```python
from build123d import *

# Parameters (mm, degrees)
SKETCH2_R           = 9.7
SKETCH2_R_2         = 6.75
SKETCH2_W           = 4.5
SKETCH2_H           = 14.8
SKETCH2_W_2         = 16.6
SKETCH2_H_2         = 4.4
BOSS_EXTRUDE1_DEPTH = 3.7
FILLET1_R           = 15
FILLET2_R           = 25
FILLET3_R           = 10


with BuildPart() as part:
    # Sketch2 → Boss-Extrude1 (new body)
    with BuildSketch(Plane.XY):
        Polygon((-66.408376963, -37.473298429), (-66.408376963, 53.126701571), (-57.108376963, 53.126701571), (-39.206701064, 34.826701571), (48.193298936, 34.826701571), (65.490462758, 53.699118578), (74.790462758, 53.699118578), (74.790462758, -29.400881422), align=None)
        with Locations((55.690462758, -8.957731732)):
            Circle(SKETCH2_R, mode=Mode.SUBTRACT)
        with Locations((-42.158376963, -6.98947646)):
            Circle(SKETCH2_R_2, mode=Mode.SUBTRACT)
        with Locations((-60.558376963, 35.726701571)):
            Rectangle(SKETCH2_W, SKETCH2_H, mode=Mode.SUBTRACT)
        with Locations((70.815419874, 35.726701571)):
            Rectangle(SKETCH2_W, SKETCH2_H, mode=Mode.SUBTRACT)
        with Locations((-11.433419848, 23.626701571)):
            Rectangle(SKETCH2_W_2, SKETCH2_H_2, mode=Mode.SUBTRACT)
        with Locations((21.690462758, 23.626701571)):
            Rectangle(SKETCH2_W_2, SKETCH2_H_2, mode=Mode.SUBTRACT)
        with BuildLine():
            Line((7.428521455, -3.001867406), (7.428521455, -25.037089926))
            ThreePointArc((7.428521455, -25.037089926), (5.128521455, -27.337089926), (2.828521455, -25.037089926))
            Line((2.828521455, -25.037089926), (2.828521455, -3.001867406))
            ThreePointArc((2.828521455, -3.001867406), (5.128521455, -0.701867406), (7.428521455, -3.001867406))
        make_face(mode=Mode.SUBTRACT)
    extrude(amount=BOSS_EXTRUDE1_DEPTH)

    # Fillet1
    fillet1_edges = [part.edges().sort_by_distance(p)[0] for p in [
        (74.790462758, -29.400881422, 1.85),
    ]]
    fillet(fillet1_edges, radius=FILLET1_R)

    # Fillet2
    fillet2_edges = [part.edges().sort_by_distance(p)[0] for p in [
        (-66.408376963, -37.473298429, 1.85),
    ]]
    fillet(fillet2_edges, radius=FILLET2_R)

    # Fillet3
    fillet3_edges = [part.edges().sort_by_distance(p)[0] for p in [
        (-39.206701064, 34.826701571, 1.85),
        (48.193298936, 34.826701571, 1.85),
    ]]
    fillet(fillet3_edges, radius=FILLET3_R)


solid = part.part
```
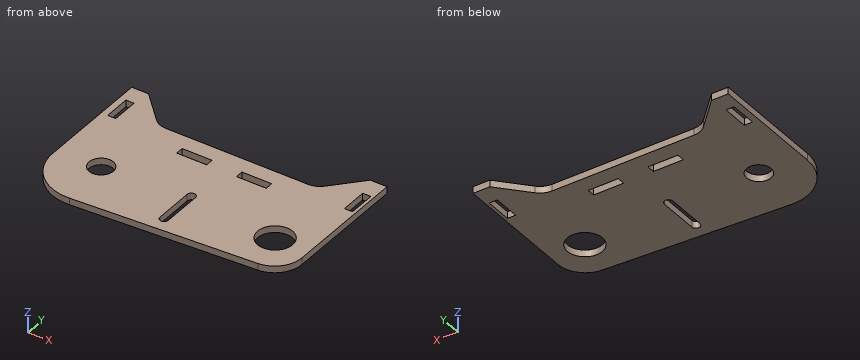
Geometry: final body of the model. Coordinates: model frame, mm. Coordinates: 2 decimals unless noted, no trailing zeros. Order: outer loops, then holes, each group sorted by start corner. A loop starts at its lowest first (then second) coordinate and runs counter-clockwise, first axis right, second up.
Item 1: Contact query for flat-ended pins moving along their axis: P1, Ø1.8, axis at x = 18.5, z = 2, coming from the +Y side; P2, Ø10, axis at x = -12, y = 40, coming from the -Z side. Output: stop coordinate, or through.
Answer:
P1: stops at y = 34.83
P2: passes through
Item 2: Section query B-B (x = 17). Output: boundary loops of the cut face in (y, z), then the cut area to 3 significant figures.
Answer:
outline: (-32.7, 0) - (21.43, 0) - (21.43, 3.7) - (-32.7, 3.7) - close; (25.83, 0) - (34.83, 0) - (34.83, 3.7) - (25.83, 3.7) - close
area: 234 mm2
Item 3: Section query D-D (x = 37). Output: boundary loops of the cut face in (y, z), then the cut area to 3 significant figures.
Answer:
outline: (-31.56, 0) - (34.83, 0) - (34.83, 3.7) - (-31.56, 3.7) - close
area: 246 mm2
Item 4: Material intervals for line 1 along X through (y, z) = (-12.5, 1.45); line 2 along X through (y, z) = (-4.5, 0.6); line 3 along Y through (x, z) = (-23, 1.5), sorted ascending.
Answer:
line 1: x = -66.36 to -46.06, -38.26 to 2.83, 7.43 to 46.66, 64.72 to 74.79
line 2: x = -66.41 to -48.43, -35.88 to 2.83, 7.43 to 47.08, 64.31 to 74.79
line 3: y = -34.99 to 34.83
Item 5: Section query A-A (y = -20). Output: boundary loops of the cut face in (x, z).
Answer:
outline: (-64.73, 0) - (2.83, 0) - (2.83, 3.7) - (-64.73, 3.7) - close; (7.43, 0) - (74.01, 0) - (74.01, 3.7) - (7.43, 3.7) - close
Item 6: Section query C-C (z = 1.5). State how many separate pieces and enclosed holes the cut face has, then the cut area to 3 significant figures.
Answer:
separate pieces: 1
enclosed holes: 7
area: 9,290 mm2
